from build123d import *

# Parameters (mm, degrees)
AXIAL_PROFILE_MM_W     = 5
AXIAL_PROFILE_MM_H     = 20.8
AXIAL_HOLES_DEPTH      = 155.634051877
AXIAL_HOLES_DEPTH_BACK = 155.634051877
SKETCH2_R              = 5.2
SKETCH2_R_2            = 2.4
SKETCH2_R_3            = 1.65
SKETCH2_R_4            = 2.85


with BuildPart() as part:
    # Axial profile (mm) → Full revolution (revolve)
    with BuildSketch(Plane.XY, mode=Mode.PRIVATE) as full_revolution_sk:
        with Locations((146.2, 19.6)):
            Rectangle(AXIAL_PROFILE_MM_W, AXIAL_PROFILE_MM_H)
    revolve(full_revolution_sk.sketch.rotate(Axis((-110, 0, 0), (1, 0, 0)), 90), axis=Axis((-110, 0, 0), (1, 0, 0)))

    # Sketch2 → Axial holes (cut, two sides: drawn at the far end of the back side and taken through both)
    with BuildSketch(Plane(origin=(0, 0, 0), x_dir=(0, 0, -1), z_dir=(1, 0, 0)).offset(-AXIAL_HOLES_DEPTH_BACK)):
        with Locations((0, 21)):
            Circle(SKETCH2_R)
        with Locations((-14.849242405, 14.849242405)):
            Circle(SKETCH2_R)
        with Locations((-21, 0)):
            Circle(SKETCH2_R)
        with Locations((-14.849242405, -14.849242405)):
            Circle(SKETCH2_R)
        with Locations((0, -21)):
            Circle(SKETCH2_R)
        with Locations((14.849242405, -14.849242405)):
            Circle(SKETCH2_R)
        with Locations((21, 0)):
            Circle(SKETCH2_R)
        with Locations((14.849242405, 14.849242405)):
            Circle(SKETCH2_R)
        with Locations((-1.977382665, 12.848733704)):
            Circle(SKETCH2_R_2)
        with Locations((-7.687206041, 10.483647423)):
            Circle(SKETCH2_R_2)
        with Locations((-12, 0)):
            Circle(SKETCH2_R_3)
        with Locations((6, -10.392304845)):
            Circle(SKETCH2_R_3)
        with Locations((6, 10.392304845)):
            Circle(SKETCH2_R_3)
        with Locations((-29.4, 0)):
            Circle(SKETCH2_R_4)
        with Locations((14.7, -25.461146871)):
            Circle(SKETCH2_R_4)
        with Locations((14.7, 25.461146871)):
            Circle(SKETCH2_R_4)
    extrude(amount=AXIAL_HOLES_DEPTH + AXIAL_HOLES_DEPTH_BACK, mode=Mode.SUBTRACT)


solid = part.part
Design review of the part built by this model. Coordinates are the model's own, in mm. Coordinates: 2 decimals unless noted, no trailing zeros. Order: outer loops, then holes, each group sorted by start corner. A loop starts at its lowest first (then second) coordinate and runs counter-clockwise, first axis right, second up.
Item 1: Take a section at B-B, the plane z = 12. Write out the cut boundary in (x, y).
Item 2: The part is to be moulded in two halves that separate along Z. For faces 1 (the cylindrical face through (146.23, 26.18, 14.65)), 2 (the cylindrical face through (146.165, 23.028, -13.215)), 3 (the cylindrical face through (146.165, -22.959, -13.335)), 4 (the flat face through (143.7, -7, 7)), say which applies: pulls with the +Z half, pulls with the -Z half, needs draft (parallel to the pull), parting line crosses it, or undercut.
Item 3: Take a section at C-C, the plane x = 144.7. Count the separate pieces of the cut face and the enclosed holes in it, then the cut area to 3 significant figures.
Item 4: For pin 1 Ø8.5 at (y, z) = (-14.85, -14.85) entering from +X; pin 2 Ø1.5 at (x, z) = (147, 23) entering from -Y; pin 3 Ø1 at (x, z) = (145, 5.5) entering from +Y; pin 4 Ø2 at (x, y) = (146, 19) entering from -Z, all flat-tipped, find the tip position at first contact; note any pin that passes through.
Item 5: Take a section at A-A, the plane y = 21. Write out the cut boundary in (x, z).
Item 6: For line 1 (Y direction, x = 147.65, z = 6.5); line 2 (Y direction, x = 145, z = 0); line 3 (Z direction, x = 146.35, y = 4), list the stretches that pass through material, from the lowest coordinate up.
The answers:
1. outline: (143.7, -27.5) - (148.7, -27.5) - (148.7, -19.2) - (143.7, -19.2) - close; (143.7, -10.5) - (148.7, -10.5) - (148.7, -1.65) - (143.7, -1.65) - close; (143.7, 1.65) - (148.7, 1.65) - (148.7, 10.5) - (143.7, 10.5) - close; (143.7, 19.2) - (148.7, 19.2) - (148.7, 27.5) - (143.7, 27.5) - close
2. face 1: parting line crosses it
2. face 2: undercut
2. face 3: undercut
2. face 4: needs draft
3. separate pieces: 1
3. enclosed holes: 14
3. area: 1,770 mm2
4. pin 1: passes through
4. pin 2: stops at y = -20.12
4. pin 3: stops at y = 29.58
4. pin 4: stops at z = -24
5. outline: (143.7, -21.42) - (148.7, -21.42) - (148.7, -5.2) - (143.7, -5.2) - close; (143.7, 5.2) - (148.7, 5.2) - (148.7, 21.42) - (143.7, 21.42) - close
6. line 1: y = -29.29 to -6.51, 6.51 to 8.4, 12.57 to 29.29
6. line 2: y = -30 to -26.2, -15.8 to -9.2, 9.2 to 11.49, 14.21 to 15.8, 26.2 to 30
6. line 3: z = -29.73 to -24.32, -17.68 to -8.28, 8.28 to 17.68, 24.32 to 29.73
